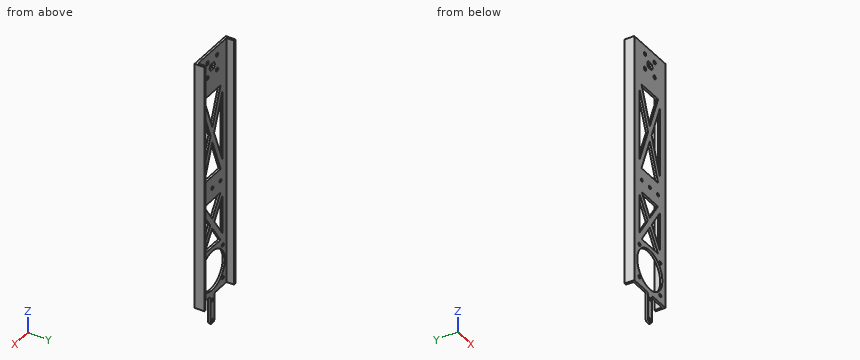
from build123d import *

# Parameters (mm, degrees)
SKETCH_2_W           = 42
SKETCH_2_H           = 46
SKETCH_2_R           = 18.5
EXTRUDE_1_DEPTH      = 2
SKETCH_3_R           = 1.6
CUT_EXTRUDE_1_DEPTH  = 32.208973069
SKETCH_4_W           = 42
SKETCH_4_H           = 187
EXTRUDE_2_DEPTH      = 2
SKETCH_7_W           = 6
SKETCH_7_H           = 27.05
SKETCH_7_R           = 1.5
EXTRUDE_4_DEPTH      = 2
FILLET_3_R           = 2
SKETCH_5_R           = 1.75
CUT_EXTRUDE_2_DEPTH  = 212.056864375
SKETCH_9_W           = 30
SKETCH_9_H           = 80
SKETCH_9_H_2         = 45
CUT_EXTRUDE_4_DEPTH  = 212.056864375
EXTRUDE_5_DEPTH      = 2
EXTRUDE_6_DEPTH      = 2
EXTRUDE_7_DEPTH      = 7
EXTRUDE_7_DEPTH_BACK = 2
SKETCH_13_W          = 2
SKETCH_13_H          = 233
SKETCH_15_R          = 1.5
CUT_EXTRUDE_5_DEPTH  = 212.371710501


with BuildPart() as part:
    # Sketch 2 → Extrude 1 (new body)
    with BuildSketch(Plane(origin=(0, 0, 0), x_dir=(1, 0, 0), z_dir=(0, 1, 0))):
        Rectangle(SKETCH_2_W, SKETCH_2_H)
        with Locations(Location((0, 0, 0), (0, 0, 270))):
            Circle(SKETCH_2_R, mode=Mode.SUBTRACT)
    extrude(amount=EXTRUDE_1_DEPTH)

    # Sketch 3 → Cut-Extrude 1 (cut, through all)
    with BuildSketch(Plane(origin=(0, 2, 0), x_dir=(1, 0, 0), z_dir=(0, 1, 0))):
        with Locations(Location((-15.5, 15.5, 0), (0, 0, 270))):
            Circle(SKETCH_3_R)
        with Locations(Location((15.5, 15.5, 0), (0, 0, 270))):
            Circle(SKETCH_3_R)
        with Locations(Location((-15.5, -15.5, 0), (0, 0, 270))):
            Circle(SKETCH_3_R)
        with Locations(Location((15.5, -15.5, 0), (0, 0, 270))):
            Circle(SKETCH_3_R)
    extrude(amount=-CUT_EXTRUDE_1_DEPTH, mode=Mode.SUBTRACT)

    # Sketch 4 → Extrude 2 (add)
    with BuildSketch(Plane(origin=(0, 2, 0), x_dir=(1, 0, 0), z_dir=(0, 1, 0))):
        with Locations((0, -116.5)):
            Rectangle(SKETCH_4_W, SKETCH_4_H)
    extrude(amount=-EXTRUDE_2_DEPTH)

    # Sketch 7 → Extrude 4 (add)
    with BuildSketch(Plane(origin=(0, 2, 0), x_dir=(1, 0, 0), z_dir=(0, 1, 0))):
        with Locations((0, 36.525)):
            Rectangle(SKETCH_7_W, SKETCH_7_H)
        with Locations(Location((0, 47.4, 0), (0, 0, 270))):
            Circle(SKETCH_7_R, mode=Mode.SUBTRACT)
        with Locations(Location((0, 28, 0), (0, 0, 270))):
            Circle(SKETCH_7_R, mode=Mode.SUBTRACT)
    extrude(amount=-EXTRUDE_4_DEPTH)

    # Fillet 3
    fillet_3_edges = [part.edges().sort_by_distance(p)[0] for p in [
        (3, 1, -23),
        (-3, 1, -23),
        (-3, 1, -50.05),
        (3, 1, -50.05),
    ]]
    fillet(fillet_3_edges, radius=FILLET_3_R)

    # Sketch 5 → Cut-Extrude 2 (cut, through all)
    with BuildSketch(Plane(origin=(0, 2, 0), x_dir=(1, 0, 0), z_dir=(0, 1, 0))):
        with Locations(Location((-7.071067812, -202.071067812, 0), (0, 0, 270))):
            Circle(SKETCH_5_R)
        with Locations(Location((7.071067812, -202.071067812, 0), (0, 0, 270))):
            Circle(SKETCH_5_R)
        with Locations(Location((-7.071067812, -187.928932188, 0), (0, 0, 270))):
            Circle(SKETCH_5_R)
        with Locations(Location((7.071067812, -187.928932188, 0), (0, 0, 270))):
            Circle(SKETCH_5_R)
        with BuildLine():
            Line((-2.156670728, -192), (2.438064686, -192))
            ThreePointArc((2.438064686, -192), (3.865767636, -195), (2.438064686, -198))
            Line((2.438064686, -198), (-2.156670728, -198))
            ThreePointArc((-2.156670728, -198), (-3.694756911, -195), (-2.156670728, -192))
        make_face()
    extrude(amount=-CUT_EXTRUDE_2_DEPTH, mode=Mode.SUBTRACT)

    # Sketch 9 → Cut-Extrude 4 (cut, through all)
    with BuildSketch(Plane(origin=(0, 2, 0), x_dir=(1, 0, 0), z_dir=(0, 1, 0))):
        with Locations((0, -130)):
            Rectangle(SKETCH_9_W, SKETCH_9_H)
        with Locations((0, -45)):
            Rectangle(SKETCH_9_W, SKETCH_9_H_2)
    extrude(amount=-CUT_EXTRUDE_4_DEPTH, mode=Mode.SUBTRACT)

    # Sketch 10 → Extrude 5 (add)
    with BuildSketch(Plane(origin=(0, 2, 0), x_dir=(1, 0, 0), z_dir=(0, 1, 0))):
        Polygon((12.919874264, -68.886750491), (-17.080125736, -23.886750491), (-12.919874264, -21.113249509), (17.080125736, -66.113249509), align=None)
        Polygon((12.659177056, -170.877808604), (-17.340822944, -90.877808604), (-12.659177056, -89.122191396), (17.340822944, -169.122191396), align=None)
    extrude(amount=-EXTRUDE_5_DEPTH)

    # Sketch 11 → Extrude 6 (add)
    with BuildSketch(Plane(origin=(0, 2, 0), x_dir=(1, 0, 0), z_dir=(0, 1, 0))):
        Polygon((-17.080125736, -66.113249509), (12.919874264, -21.113249509), (17.080125736, -23.886750491), (-12.919874264, -68.886750491), align=None)
        Polygon((-12.659177056, -170.877808604), (17.340822944, -90.877808604), (12.659177056, -89.122191396), (-17.340822944, -169.122191396), align=None)
    extrude(amount=-EXTRUDE_6_DEPTH)

    # Sketch 13 → Extrude 7 (add, two sides: drawn at the far end of the back side and taken through both)
    with BuildSketch(Plane(origin=(0, 2, 0), x_dir=(1, 0, 0), z_dir=(0, 1, 0)).offset(-EXTRUDE_7_DEPTH_BACK)):
        with Locations((22, -93.5)):
            Rectangle(SKETCH_13_W, SKETCH_13_H)
        with Locations((-22, -93.5)):
            Rectangle(SKETCH_13_W, SKETCH_13_H)
    extrude(amount=EXTRUDE_7_DEPTH + EXTRUDE_7_DEPTH_BACK)

    # Sketch 15 → Cut-Extrude 5 (cut, through all)
    with BuildSketch(Plane(origin=(0, 2, 0), x_dir=(1, 0, 0), z_dir=(0, 1, 0))):
        with Locations(Location((0, -78.75, 0), (0, 0, 270))):
            Circle(SKETCH_15_R)
        with Locations(Location((-12, -78.75, 0), (0, 0, 270))):
            Circle(SKETCH_15_R)
        with Locations(Location((12, -78.75, 0), (0, 0, 270))):
            Circle(SKETCH_15_R)
    extrude(amount=-CUT_EXTRUDE_5_DEPTH, mode=Mode.SUBTRACT)


solid = part.part
Work out the finished part from the listing and answer in its coordinate system (mm). Give positions to 0.01 mm unless a question says otherwise; leave off trailing zeros. Loops run counter-clockwise (first coordinate to the right, second up) from the corner with the lowest first, then second, coordinate; pieces in that order, holes last. Notation, with made-up numbers: (89.25, 63.5) -> (114.25, 63.5) arc R22 cw to (114.25, 98.5) -> close; hole circle Ø7 at (25, 32). An arc over 180 degrees is marked (long way). Use a Markdown table: item, result. Add a question column.
1. Find the intervals of material crossed by probe 1 along X at (y, z) = (0.7, 78.75); probe 2 along X at (y, z) = (7.5, 102); probe 3 along X at (y, z) = (0.5, 33), in increasing order.
2. Section A-A on y = 4.5 is taken. Determine the outline of the cut face in (x, z).
3. Section B-B on z = 155 is taken. Determine the outline of the cut face in (x, y) (3 decimals), and give its area (3 significant figures).
4. Flat-ended cylindrical pins translate along their axes: pin 1 Ø4 at (x, z) = (0, -47.4) entering from +Y; pin 2 Ø2 at (x, y) = (-4.5, 1) entering from -Z; pin 3 Ø2.5 at (x, z) = (-15.5, 15.5) entering from +Y; pin 4 Ø1.6 at (y, z) = (1, -37) entering from -X. Find the tip coordinate at first contact, or state that the pin passes through.
5. Section C-C on z = 33 is taken. Determine the outline of the cut face in (x, y), and give its area (3 significant figures).
Results below:
| question | item | result |
|---|---|---|
| 1 | probe 1 | x = -23 to -13.5, -10.5 to -1.5, 1.5 to 10.5, 13.5 to 23 |
| 1 | probe 2 | x = -23 to -21, 21 to 23 |
| 1 | probe 3 | x = -23 to -15, -11 to -5, 5 to 11, 15 to 23 |
| 2 | outline | (-23, -23) -> (-21, -23) -> (-21, 210) -> (-23, 210) -> close; (21, -23) -> (23, -23) -> (23, 210) -> (21, 210) -> close |
| 3 | outline | (-23, 0) -> (-15, 0) -> (-15, 2) -> (-21, 2) -> (-21, 9) -> (-23, 9) -> close; (-12.045, 0) -> (-6.705, 0) -> (-6.705, 2) -> (-12.045, 2) -> close; (6.705, 0) -> (12.045, 0) -> (12.045, 2) -> (6.705, 2) -> close; (15, 0) -> (23, 0) -> (23, 9) -> (21, 9) -> (21, 2) -> (15, 2) -> close |
| 3 | area | 81.4 mm^2 |
| 4 | pin 1 | stops at y = 2 |
| 4 | pin 2 | stops at z = -23.68 |
| 4 | pin 3 | passes through |
| 4 | pin 4 | stops at x = -3 |
| 5 | outline | (-23, 0) -> (-15, 0) -> (-15, 2) -> (-21, 2) -> (-21, 9) -> (-23, 9) -> close; (-11, 0) -> (-5, 0) -> (-5, 2) -> (-11, 2) -> close; (5, 0) -> (11, 0) -> (11, 2) -> (5, 2) -> close; (15, 0) -> (23, 0) -> (23, 9) -> (21, 9) -> (21, 2) -> (15, 2) -> close |
| 5 | area | 84.0 mm^2 |
